Print and shaded views of the part. All mm, measured from the part's lowest x, y and z. A direction names the side the tool comes from. Round coordinates to 2 decimals unless told otherwise and drop trailing zeros. Order: outer loops, then holes, each group sorted by start corner. A loop starts at its lowest first (then second) coordinate and runs counter-clockwise, first axis right, second up. Notation, with made-up numbers: (58, -1) -> (72, -1) arc R12 cw to (72, 15) -> close; hole circle Ø5 at (31.25, -34). An arc over 180 degrees is marked (long way). Answer as CSV lines item,"result". Start each with the question number.
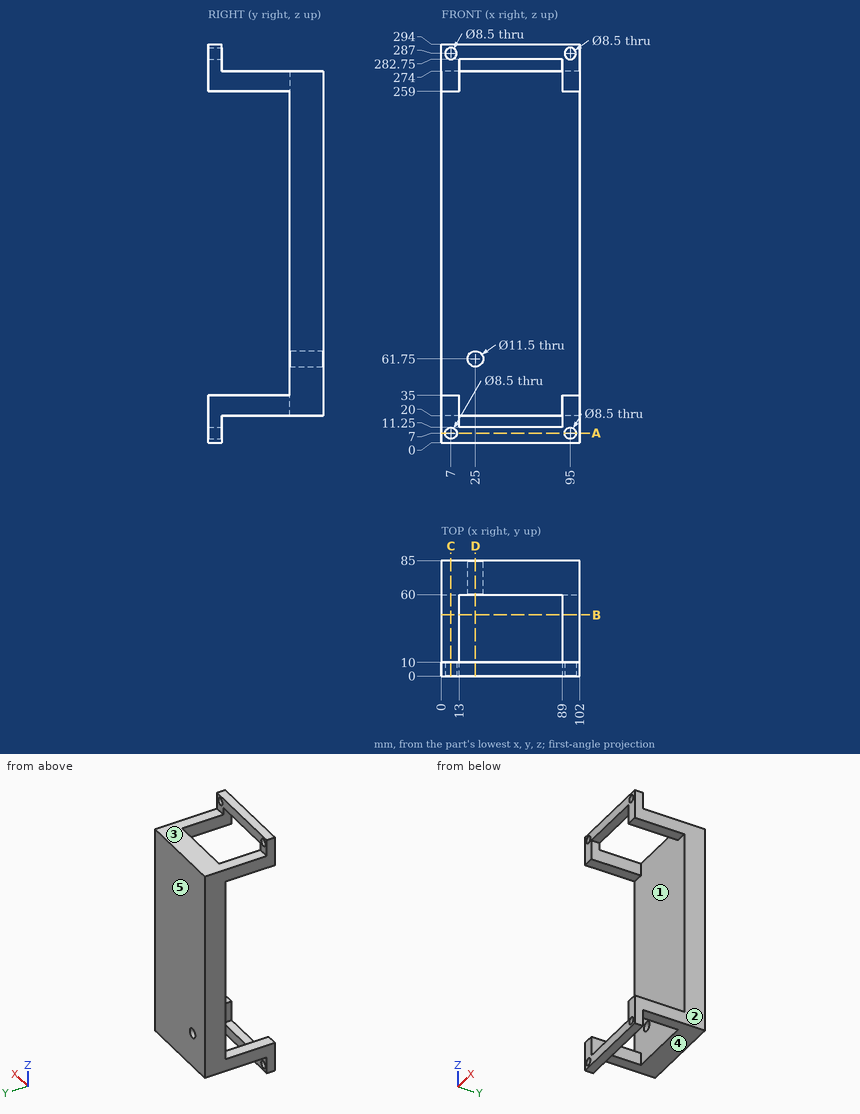
Item 1: Band-saw the part on B-B, the plane y = 45. Give the cut face in (x, z).
Item 2: Band-saw the part on D-D, the plane x = 25. Give the cut face in (y, z).
Item 3: Mould opens along Z. For the marked faces 1, 2 and 3 say: released by +Z, released by -Z, zero draft, split by the parting line, or undercut.
Item 4: Band-saw the part on C-C, the plane x = 7. Give the cut face in (y, z), and give its area (3 significant figures).
Item 5: Band-saw the part on A-A, the plane z = 7. Give the cut face in (x, y), and give its area (3 significant figures).
Item 6: Probe line 1 (X direction, y = 5.75, z = 7); line 2 (Z direction, x = 95, y = 8); line 3 (Y direction, x = 34, z = 118). List the from-to ranges inside material, lowest first.
Item 7: Pin check, flat tips, straight feed: pin 1 (10.5 mm diameter, centred on x = 9.5, y = 26, fed in from +Z); pin 2 (2 mm diameter, centred on x = 91.5, z = 163, fed in from -Y); pin 3 (22.5 mm diameter, centred on x = 52.5, y = 65, fed in from -Z). Stop position of each tip, or through.
Item 8: Tool access for the marked faces 4 and 5: list every direction of +Z, -Z, +X, -X, +Y, -Y with a clear straight run to the whole face (end or side of a thin tool).
Values:
1,outline,"(0, 20) -> (13, 20) -> (13, 35) -> (0, 35) -> close; (0, 259) -> (13, 259) -> (13, 274) -> (0, 274) -> close; (89, 20) -> (102, 20) -> (102, 35) -> (89, 35) -> close; (89, 259) -> (102, 259) -> (102, 274) -> (89, 274) -> close"
2,outline,"(0, 0) -> (10, 0) -> (10, 11.25) -> (0, 11.25) -> close; (0, 282.75) -> (10, 282.75) -> (10, 294) -> (0, 294) -> close; (60, 20) -> (85, 20) -> (85, 56) -> (60, 56) -> close; (60, 67.5) -> (85, 67.5) -> (85, 274) -> (60, 274) -> close"
3,face 1,"undercut"
3,face 2,"zero draft"
3,face 3,"released by +Z"
4,outline,"(0, 0) -> (10, 0) -> (10, 2.75) -> (0, 2.75) -> close; (0, 11.25) -> (10, 11.25) -> (10, 20) -> (85, 20) -> (85, 274) -> (10, 274) -> (10, 282.75) -> (0, 282.75) -> (0, 259) -> (60, 259) -> (60, 35) -> (0, 35) -> close; (0, 291.25) -> (10, 291.25) -> (10, 294) -> (0, 294) -> close"
4,area,"8,380 mm²"
5,outline,"(0, 0) -> (2.75, 0) -> (2.75, 10) -> (0, 10) -> close; (11.25, 0) -> (90.75, 0) -> (90.75, 10) -> (11.25, 10) -> close; (99.25, 0) -> (102, 0) -> (102, 10) -> (99.25, 10) -> close"
5,area,"850 mm²"
6,line 1,"0 to 2.75, 11.25 to 90.75, 99.25 to 102"
6,line 2,"0 to 2.75, 11.25 to 35, 259 to 282.75, 291.25 to 294"
6,line 3,"60 to 85"
7,pin 1,"z = 274"
7,pin 2,"y = 60"
7,pin 3,"z = 20"
8,face 4,"-Z, +X, -X, +Y"
8,face 5,"+Z, -Z, +X, -X, +Y"
